```python
from build123d import *

# Parameters (mm, degrees)
EXTRUDE_1_DEPTH = 19


with BuildPart() as part:
    # Эскиз1 → Вытянуть1 (new body)
    with BuildSketch(Plane.XY):
        with BuildLine():
            Line((-5.996779713, 0.196552972), (-4.569380805, 90.185232995))
            Line((-4.569380805, 90.185232995), (-14.032554186, 106.456860521))
            ThreePointArc((-14.032554186, 106.456860521), (-16.738501903, 116.052970381), (-14.475382715, 125.763056325))
            Line((-14.475382715, 125.763056325), (-7.67310326, 138.800500371))
            ThreePointArc((-7.67310326, 138.800500371), (-5.665255915, 144.834300954), (-5.652980092, 151.193392849))
            Line((-5.652980092, 151.193392849), (-8.669783562, 170.161558564))
            ThreePointArc((-8.669783562, 170.161558564), (-3.453313414, 175.494197645), (3.037538011, 171.817589403))
            Line((3.037538011, 171.817589403), (6.382811975, 150.78416394))
            ThreePointArc((6.382811975, 150.78416394), (6.370536152, 144.425072045), (4.362688807, 138.391271463))
            Line((4.362688807, 138.391271463), (-2.373176384, 125.481118902))
            ThreePointArc((-2.373176384, 125.481118902), (-4.636295572, 115.771032958), (-1.930347854, 106.174923097))
            Line((-1.930347854, 106.174923097), (7.483697652, 89.987769398))
            Line((7.483697652, 89.987769398), (6, 0))
            Line((6, 0), (-5.996779713, 0.196552972))
        make_face()
    extrude(amount=EXTRUDE_1_DEPTH)


solid = part.part
```
Input: part model. Units: mm. Frame: model coordinates. A direction names the side the tool comes from. Give positions to 0.01 mm unless a question says otherwise; leave off trailing zeros. Order: outer loops, then holes, each group sorted by start corner. A loop starts at its lowest first (then second) coordinate and runs counter-clockwise, first axis right, second up. Notation, with made-up numbers: M 28.25,10.5 L 72.25,10.5 A14 cw 72.25,23.5 Z; hole C -31,56.5 d11. An arc over 180 degrees is marked long. One line per question, with ' | ' between items. Start each with the question number.
1. Material intervals for probe 1 along Y at (x, z) = (-1, 12); probe 2 along Y at (x, z) = (-0.5, 5.5); probe 3 along X at (y, z) = (61.5, 12.75), sorted ascending. Write a range as [from, to].
2. Section query A-A (x = 1). Return the cut outline in (y, z).
3. Pull-direction query (Y, two-part tool) for faces 3 (the face through (-7.14, 160.54, 9.37)), 4 (the face through (4.687, 161.448, 9.367)), 5 (the face through (-2, 89, 0)); classes: released by +Y, released by -Y, zero draft, split by the parting line, or undercut.
4. Section query B-B (z = 4). Return the cut outline in (x, y), and give its area (3 significant figures).
5. Section query D-D (y = 40). Return the cut outline in (x, z).
6. First-contact query: pin 1 Ø1.5 at (x, z) = (-7.5, 13) entering from +Y; pin 2 Ø8 at (y, z) = (129.5, 13) entering from -X; pin 3 Ø10 at (x, y) = (-10.5, 78) entering from -Z; pin 4 Ø4 at (y, z) = (50, 6.5) entering from +X. Flat tips, straight axial feed; report the tip coordinate or a pass-through.
7. Section query C-C (y = 71.5). Return the cut outline in (x, z), and give its area (3 significant figures).
8. Access query for faces 1 (the face through (-3.56, 175.48, 9.37)), 2 (the face through (1.042, 132.027, 9.367)). Directions: +Z, -Z, +X, -X, +Y, -Y. A direction counts if a zero-diameter tool reaches every point of the face in a straight line with its end or side. Return the directions, or none.
Here are the results:
1) probe 1: [0.11, 104.58], [128.11, 175.34] | probe 2: [0.11, 103.72], [129.07, 175.18] | probe 3: [-5.02, 7.01]
2) outline: M 0.08,0 L 101.14,0 L 101.14,19 L 0.08,19 Z; M 131.95,0 L 174.39,0 L 174.39,19 L 131.95,19 Z
3) face 3: undercut | face 4: released by +Y | face 5: zero draft
4) outline: M -14.48,125.76 A20 ccw -14.03,106.46 L -4.57,90.19 L -6,0.2 L 6,0 L 7.48,89.99 L -1.93,106.17 A20 cw -2.37,125.48 L 4.36,138.39 A20 ccw 6.38,150.78 L 3.04,171.82 A6.12 ccw -8.67,170.16 L -5.65,151.19 A20 cw -7.67,138.8 Z | area: 2,100 mm²
5) outline: M -5.37,0 L 6.66,0 L 6.66,19 L -5.37,19 Z
6) pin 1: y = 173.93 | pin 2: x = -14.61 | pin 3: through | pin 4: x = 6.86
7) outline: M -4.87,0 L 7.18,0 L 7.18,19 L -4.87,19 Z | area: 229 mm²
8) face 1: +Z, -Z, +Y | face 2: +Z, -Z, +X
